Can you work these out from the drawing? Everything is in mm from the part's minimum corner. A direction names the side the tool comes from. Give positions to 0.01 mm unless a question says otherwise; leave off trailing zeros. Order: outer loops, then holes, each group sorted by start corner. A loop starts at its lowest first (then second) coordinate and runs counter-clockwise, first axis right, second up. Notation, with made-up numbers: (-7.5, -10.75) - (46.5, -10.75) arc R16 ccw to (46.5, 20.25) - close; hole circle Ø1 at (9, -36.5). An arc over 180 degrees is marked (long way). One line per question, with ' | ' between items.
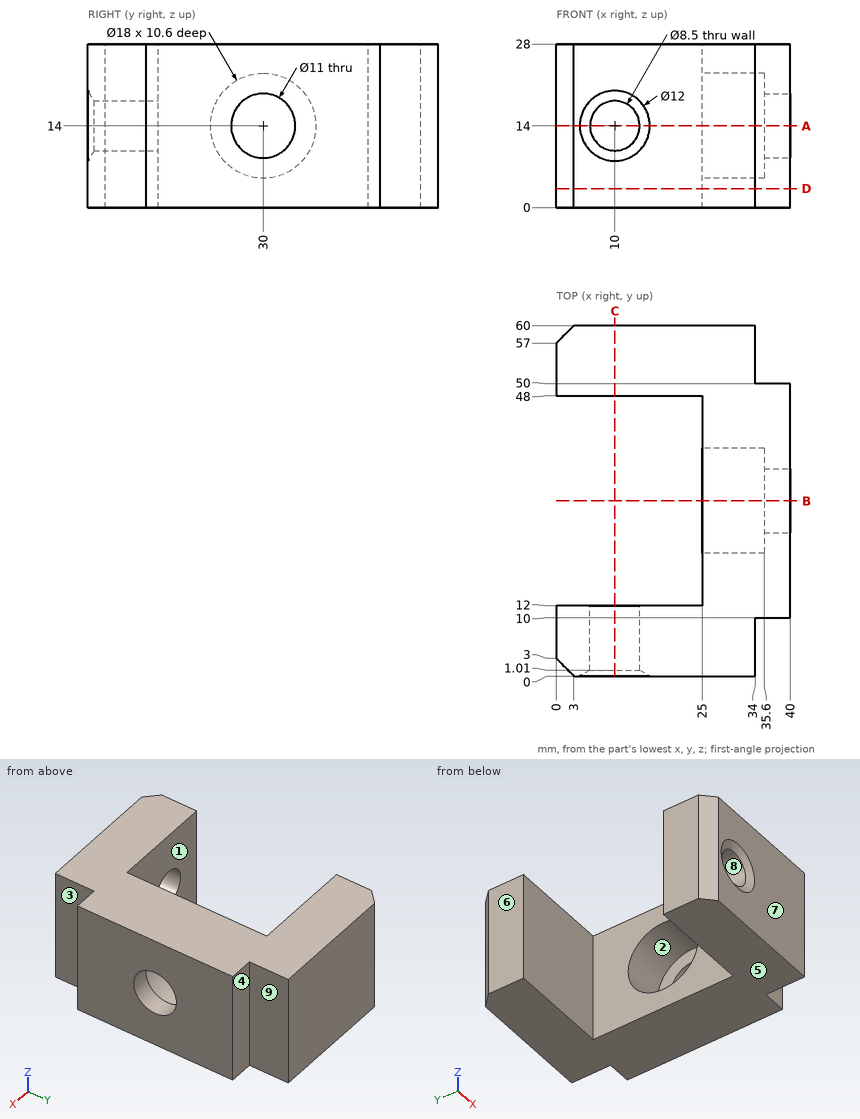
(1) Imagine slicing it at D-D (z = 3.25). List the corners of the cut face in (x, y) for me.
Answer below:
outline: (0, 3) - (3, 0) - (34, 0) - (34, 10) - (40, 10) - (40, 50) - (34, 50) - (34, 60) - (3, 60) - (0, 57) - (0, 48) - (25, 48) - (25, 12) - (0, 12) - close
(2) Imagine slicing it at A-A (z = 14). List the corners of the cut face in (x, y) for me.
Answer below:
outline: (0, 3) - (3, 0) - (4, 0) - (5.75, 1.01) - (5.75, 12) - (0, 12) - close; (0, 48) - (25, 48) - (25, 39) - (35.6, 39) - (35.6, 35.5) - (40, 35.5) - (40, 50) - (34, 50) - (34, 60) - (3, 60) - (0, 57) - close; (14.25, 1.01) - (16, 0) - (34, 0) - (34, 10) - (40, 10) - (40, 24.5) - (35.6, 24.5) - (35.6, 21) - (25, 21) - (25, 12) - (14.25, 12) - close
(3) Will these pins go through, and if not, where does the flat tip stop? pin 1 (14.5 mm diameter, centred on y = 30, z = 14, fed in from -X); pin 2 (3 mm diameter, centred on x = 37, z = 10.5, fed in from +Y); pin 3 (3 mm diameter, centred on x = 38.5, z = 15.5, fed in from -Y); pin 4 (5 mm diameter, centred on x = 19.5, y = 10.5, fed in from -Z).
Answer below:
pin 1: x = 35.6 | pin 2: y = 50 | pin 3: y = 10 | pin 4: z = 0
(4) If we mould it in two halves opening along X, with no side actions, what happens to the marked faces 6, 7, 8 and 9? For each: released by +X, released by -X, zero draft, split by the parting line, or undercut.
Answer below:
face 6: released by -X | face 7: zero draft | face 8: undercut | face 9: released by +X
(5) Imagine slicing it at B-B (y = 30). List the corners of the cut face in (x, z) for me, and give its area (3 significant figures).
Answer below:
outline: (25, 0) - (40, 0) - (40, 8.5) - (35.6, 8.5) - (35.6, 5) - (25, 5) - close; (25, 23) - (35.6, 23) - (35.6, 19.5) - (40, 19.5) - (40, 28) - (25, 28) - close | area: 181 mm^2
(6) On a 3-axis mill with a long thin cutter (end or side, diameter ignored), from which of +Z, -Z, +X, -X, +Y, -Y can I reach the whole of each face in a straight line? I mean the marked faces 1, 2, 3, 4 and 5. Say none if no direction works.
Answer below:
face 1: +Z, -Z, -X | face 2: -X | face 3: +Z, -Z, +X, -Y | face 4: +Z, -Z, +X, +Y | face 5: -Z, +X, -X, +Y, -Y
(7) If I drill on line 1 (X direction, y = 3.75, z = 14); line 2 (Y direction, x = 3, z = 8); line 3 (Z direction, x = 10, y = 9), over which ranges is the centre line in solid material (lowest first)?
Answer below:
line 1: 0 to 5.75, 14.25 to 34 | line 2: 0 to 12, 48 to 60 | line 3: 0 to 9.75, 18.25 to 28
(8) Imagine slicing it at C-C (x = 10). List the corners of the cut face in (y, z) for me.
Answer below:
outline: (0, 0) - (12, 0) - (12, 9.75) - (1.01, 9.75) - (0, 8) - close; (0, 20) - (1.01, 18.25) - (12, 18.25) - (12, 28) - (0, 28) - close; (48, 0) - (60, 0) - (60, 28) - (48, 28) - close
